For this review, take the finished solid that the model builds, in its own axes (mm). Face numbers are marked on the shaded views. A direction names the side the tool comes from. Coordinates: 2 decimals unless noted, no trailing zeros. Loops run counter-clockwise (first coordinate to the right, second up) from the corner with the lowest first, then second, coordinate; pieces in that order, holes last. Notation, with made-up numbers: M 70,85.5 L 106,85.5 A25 cw 106,105.5 Z; hole C 39,5.5 d8. An arc over 180 degrees is marked long. Answer as a JSON object with one key per item and string values. Group by question number.
Item 1: Add section B-B (y = -3.5). State the section outline as (x, z) points, then the cut area to 3 significant figures.
Item 2: Add section D-D (z = 17.25). State the section outline as (x, y) points, then the cut area to 3 significant figures.
Item 3: Wall thickness on L1, parallel to Y at x = -23, z = 3; L2, parallel to X at y = -5.75, z = 3.75; L3, parallel to Z at x = 22, y = -14.5: over which ranges is each line inside the solid? List them lowest first. Write a range as from..to.
Item 4: Mouldability with a two-part tool opening along X and no side actions: class the marked faces 4, 5, 6 and 7 as +X half, -X half, draft (parallel to the pull), parting line (faces both ways), or undercut.
Item 5: Tool access review of the marked faces 1, 2 and 3: name each direction out of +Z, -Z, +X, -X, +Y, -Y from which nothing blocks a thin tool from reaching the whole face with its end or side.
Item 6: Add section C-C (z = 11.5). Count the separate pieces of the cut face and the enclosed holes in it, then the cut area to 3 significant figures.
Item 7: Insertion check: pin 1 (8 mm diameter, centred on x = 19.5, y = -4.5, fed in from -Z); pin 2 (5 mm diameter, centred on y = -15, z = 21.5, fed in from +X); pin 3 (5 mm diameter, centred on y = -10, z = 21, fed in from -X); pin 4 (8.5 mm diameter, centred on x = -27, y = -8.5, fed in from +Z). Each pin has a flat end and moves straight along its axis. Give the tip position at first contact, or say it passes through.
Item 8: Add section A-A (y = -10). State the section outline as (x, z) points.
from build123d import *

# Parameters (mm, degrees)
F1_DEPTH = 19.05
F3_R     = 2.54
F6_D     = 9.525


with BuildPart() as f1:
    # F0 (on Front) → F1 (new body)
    with BuildSketch(Plane.XZ):
        Polygon((-31.75, 0), (0, 0), (0, 25.4), (-12.7, 25.4), (-12.7, 12.7), (-31.75, 12.7), align=None)
    extrude(amount=F1_DEPTH)

    # F2: F1 across face


with BuildPart() as f1_1:
    add(f1.part)
    add(f1.part.mirror(Plane(origin=(0, -9.525, 12.7), x_dir=(0, 1, 0), z_dir=(1, 0, 0))))

    # F3
    f3_edges = [f1_1.edges().sort_by_distance(p)[0] for p in [
        (-31.75, -19.05, 6.35),
        (-31.75, 0, 6.35),
        (31.75, -19.05, 6.35),
        (31.75, 0, 6.35),
        (12.7, -9.525, 12.7),
        (-12.7, -9.525, 12.7),
    ]]
    fillet(f3_edges, radius=F3_R)

    # F6 (through all)
    with Locations(Plane.XY.offset(12.954)):
        with Locations((-22.9998156428, -9.2977983877), (22.9998193681, -9.2977983877)):
            Hole(F6_D / 2)


solid = f1_1.part
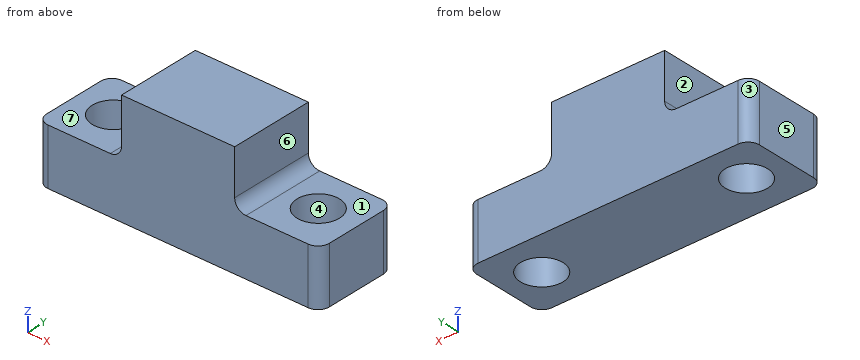
From the geometry:
{
 "1": {"outline": "M -31.75,0 L 31.75,0 L 31.75,12.7 L 15.24,12.7 A2.54 cw 12.7,15.24 L 12.7,25.4 L -12.7,25.4 L -12.7,15.24 A2.54 cw -15.24,12.7 L -31.75,12.7 Z", "area": "1,130 mm²"},
 "2": {"outline": "M -12.7,-19.05 L 12.7,-19.05 L 12.7,0 L -12.7,0 Z", "area": "484 mm²"},
 "3": {"L1": "y = -19.05..-14.06, -4.54..0", "L2": "x = -31.75..-26.18, -19.82..19.82, 26.18..31.75", "L3": "z = 0..12.7"},
 "4": {"face 4": "undercut", "face 5": "-X half", "face 6": "+X half", "face 7": "draft"},
 "5": {"face 1": "+Z, +X, +Y, -Y", "face 2": "+Z, -X, +Y, -Y", "face 3": "+Z, -Z, -X, +Y"},
 "6": {"separate pieces": "1", "enclosed holes": "2", "area": "1,060 mm²"},
 "7": {"pin 1": "stops at z = 0", "pin 2": "stops at x = 12.7", "pin 3": "stops at x = -12.7", "pin 4": "stops at z = 12.7"},
 "8": {"outline": "M -31.75,0 L -27.71,0 L -27.71,12.7 L -31.75,12.7 Z; M -18.29,0 L 18.29,0 L 18.29,12.7 L 15.24,12.7 A2.54 cw 12.7,15.24 L 12.7,25.4 L -12.7,25.4 L -12.7,15.24 A2.54 cw -15.24,12.7 L -18.29,12.7 Z; M 27.71,0 L 31.75,0 L 31.75,12.7 L 27.71,12.7 Z"}
}
